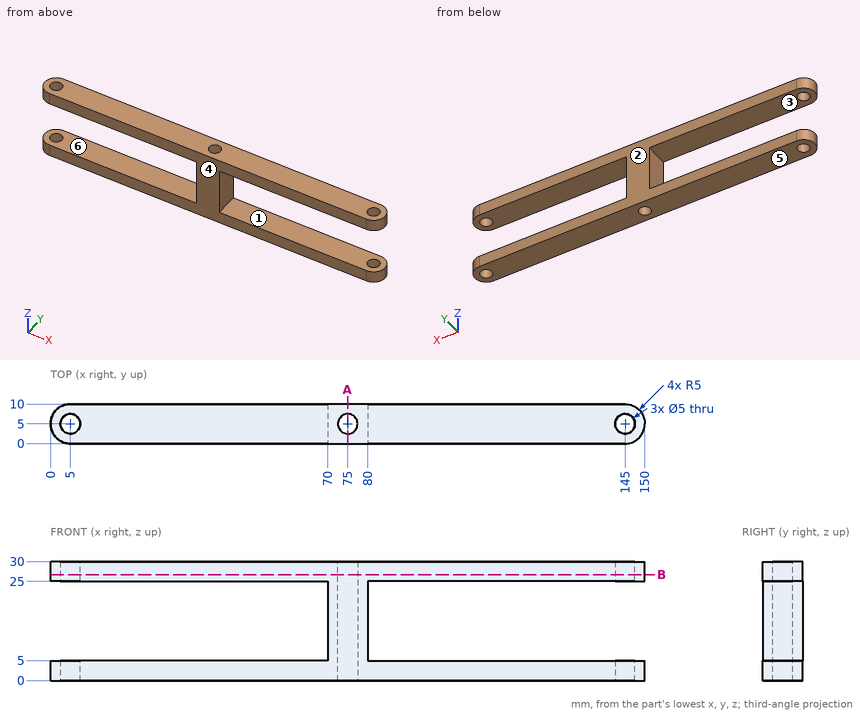
The drawing under review shows one solid part. Ordinate dimensions are in mm from its lowest x, y, z. A direction names the side the tool comes from. Round coordinates to 2 decimals unless told otherwise and drop trailing zeros. Loops run counter-clockwise (first coordinate to the right, second up) from the corner with the lowest first, then second, coordinate; pieces in that order, holes last. Notation, with made-up numbers: (-5.5, 45.5) - (8.5, 45.5) arc R6 ccw to (8.5, 56.5) - close; hole circle Ø5 at (-16, -34). An arc over 180 degrees is marked (long way). One line per item, written item: value. Start each with the question number.
1) Consider section B-B on z = 26.75. Give the number of separate pieces and of enclosed holes in the cut face, then the cut area to 3 significant figures.
2) Insertion check: pin 1 Ø3 at (y, z) = (2.5, 15.5) entering from -X; pin 2 Ø2 at (y, z) = (3, 11.5) entering from +X. Each pin has a flat end and moves straight along its axis. Give the tip position at first contact, or say it passes through.
3) Draft analysis for pull direction Z (two halves, no side actions). For the marked faces 4, 5 and 6, state which applies: +Z half, -Z half, draft (parallel to the pull), parting line (faces both ways), or undercut.
4) For the marked faces 1, 2 and 3, list the 3-axis set-ups (+Z, -Z, +X, -X, +Y, -Y) from which the entire face can be reached by the end or side of a thin tool; tool diameter is ignored.
5) To check wall thickness, follow L1, parallel to X at y = 5.25, z = 27.75; L2, parallel to Z at x = 126, y = 3.75; L3, parallel to Y at x = 145, z = 28.3. State the ranges of each line that lie inside material, in increasing order. Write a range as from..to.
6) Consider section A-A on x = 75. Give the boundary of the cut face in (y, z).
Reported:
1. separate pieces: 1
1. enclosed holes: 3
1. area: 1,420 mm^2
2. pin 1: stops at x = 70
2. pin 2: stops at x = 80
3. face 4: draft
3. face 5: -Z half
3. face 6: undercut
4. face 1: +X, +Y, -Y
4. face 2: +Z, -Z, +X, -X, +Y
4. face 3: -X, +Y, -Y
5. L1: x = 0.01..2.51, 7.49..72.51, 77.49..142.51, 147.49..149.99
5. L2: z = 0..5, 25..30
5. L3: y = 0..2.5, 7.5..10
6. outline: (0, 0) - (2.5, 0) - (2.5, 30) - (0, 30) - close; (7.5, 0) - (10, 0) - (10, 30) - (7.5, 30) - close
